Can you work these out from the model? Positions are in its coordinate system, mm. A direction names the side the tool comes from. Give positions to 0.01 mm unless a question says otherwise; leave off trailing zeros. Loops run counter-clockwise (first coordinate to the right, second up) from the corner with the lowest first, then second, coordinate; pieces in that order, holes last. Notation, with made-up numbers: (54, 37) - (88, 37) arc R11 ccw to (88, 57) - close; hole circle Ø4 at (31.25, 64.25). An arc over 180 degrees is marked (long way). Answer as a JSON object with one key per item and string values. Group by question number.
Item 1: Suppose I cut it at B-B on z = 25. Write out the boundary of the cut face in (x, y), and give its area (3 significant figures).
Item 2: Suppose I cut it at A-A on z = -9.5. Write out the boundary of the cut face in (x, y).
Item 3: Thinking about a two-plate mould opening in Y: for faces 1 (the conical face through (6.94, -6.37, 33.38)), 2 (the cylindrical face through (-2.54, -3.984, 30.685)), which applies, pulls with the +Y half, pulls with the -Y half, needs draft (parallel to the pull), parting line crosses it, or undercut?
Item 4: Please list where these lines run through material, in increasing order: L1, parallel to X at y = 0, z = 32; L2, parallel to X at y = 0, z = 28; L3, parallel to Y at x = 0, z = -12.5.
Item 5: Which directions (+Z, -Z, +X, -X, +Y, -Y) give clear straight access to the entire face, cutting with the end or side of a thin tool? Please do faces 3 (the flat face through (0, 0, 26.035)), 4 (the flat face through (0, 0, -5.842)).
Item 6: Will these pins go through, and if not, where does the flat tip stop? pin 1 (12 mm diameter, centred on x = -21.5, z = -20, fed in from +Y); pin 2 (3 mm diameter, centred on y = -20, z = -9.5, fed in from -X); pin 3 (12 mm diameter, centred on x = -4, y = -23.5, fed in from -Z).
from build123d import *

# Parameters (mm, degrees)
F0_W = 4.7244
F0_H = 9.525


# Not quite as in the source:
# - a feature names something its author has since deleted; it is built from what else it names


with BuildPart() as f1:
    # F0 (on Front) → F1 (revolve)
    with BuildSketch(Plane.XZ):
        with BuildLine():
            Line((-8.1087104998, 34.5070896671), (-22.5402639736, 16.51))
            ThreePointArc((-22.5402639736, 16.51), (-25.8838273037, -10.5200325148), (-4.6314331906, -27.5534648747))
            Line((-4.6314331906, -27.5534648747), (-1.6002, -27.8064487898))
            Line((-1.6002, -27.8064487898), (-1.6002, -5.842))
            Line((-1.6002, -5.842), (0, -5.842))
            Line((0, -5.842), (0, 0))
            Line((0, 0), (0, 3.81))
            Line((0, 3.81), (0, 16.51))
            Line((0, 16.51), (-4.7244, 16.51))
            Line((-4.7244, 16.51), (-4.7244, 26.035))
            Line((-4.7244, 26.035), (-4.7244, 35.2065371441))
            ThreePointArc((-4.7244, 35.2065371441), (-6.4260787397, 34.9028932721), (-8.1087104998, 34.5070896671))
        make_face()
        with Locations((-2.3622, 21.2725)):
            Rectangle(F0_W, F0_H)
        with BuildLine():
            Line((0, 0), (0, -5.842))
            Line((0, -5.842), (0, -25.4))
            ThreePointArc((0, -25.4), (23.0706956982, -10.625582337), (19.302328875, 16.51))
            Line((19.302328875, 16.51), (0, 16.51))
            Line((0, 16.51), (0, 3.81))
            Line((0, 3.81), (0, 0))
        make_face()
    revolve(axis=Axis((0, 0, 3.81), (0, 0, 1)))

    # F0 (on Front) → F2 (revolve)
    with BuildSketch(Plane.XZ):
        with BuildLine():
            Line((-8.1087104998, 34.5070896671), (-22.5402639736, 16.51))
            ThreePointArc((-22.5402639736, 16.51), (-25.8838273037, -10.5200325148), (-4.6314331906, -27.5534648747))
            Line((-4.6314331906, -27.5534648747), (-1.6002, -27.8064487898))
            Line((-1.6002, -27.8064487898), (-1.6002, -5.842))
            Line((-1.6002, -5.842), (0, -5.842))
            Line((0, -5.842), (0, 0))
            Line((0, 0), (0, 3.81))
            Line((0, 3.81), (0, 16.51))
            Line((0, 16.51), (-4.7244, 16.51))
            Line((-4.7244, 16.51), (-4.7244, 26.035))
            Line((-4.7244, 26.035), (-4.7244, 35.2065371441))
            ThreePointArc((-4.7244, 35.2065371441), (-6.4260787397, 34.9028932721), (-8.1087104998, 34.5070896671))
        make_face()
        with BuildLine():
            ThreePointArc((-4.6314331906, -27.5534648747), (-25.8838273037, -10.5200325148), (-22.5402639736, 16.51))
            Line((-22.5402639736, 16.51), (-29.099355663, 16.51))
            ThreePointArc((-29.099355663, 16.51), (-27.9182626522, -11.3106187202), (-5.2629922621, -27.5007555394))
            Line((-5.2629922621, -27.5007555394), (-4.6314331906, -27.5534648747))
        make_face()
        Polygon((-29.099355663, 16.51), (-22.5402639736, 16.51), (-8.1087104998, 34.5070896671), align=None)
    revolve(axis=Axis((0, 0, -12.065), (0, 0, 1)))


solid = f1.part
Worked out:
{
 "1": {"outline": "circle Ø38.39 at (0, 0)", "area": "1,160 mm2"},
 "2": {"outline": "circle Ø57.65 at (0, 0); hole circle Ø3.2 at (0, 0)"},
 "3": {"face 1": "parting line crosses it", "face 2": "undercut"},
 "4": {"L1": "x = -11.03 to -4.72, 4.72 to 11.03", "L2": "x = -15.7 to -4.72, 4.72 to 15.7", "L3": "y = -27.24 to -1.6, 1.6 to 27.24"},
 "5": {"face 3": "+Z", "face 4": "-Z"},
 "6": {"pin 1": "stops at y = 18.11", "pin 2": "stops at x = -22.38", "pin 3": "stops at z = -22.46"}
}
